Verification items for the finished model (mm, model axes). Face numbers are marked on the shaded views. Give positions to 0.01 mm unless a question says otherwise; leave off trailing zeros. Order: outer loops, then holes, each group sorted by start corner. A loop starts at its lowest first (then second) coordinate and runs counter-clockwise, first axis right, second up. Notation, with made-up numbers: (-18, 27.5) - (20, 27.5) arc R10 cw to (20, 40.5) - close; hole circle Ø5 at (-10.5, 47.5). An arc over 180 degrees is marked (long way). Answer as a JSON object with one key per item and string values. Group by question number.
(1) Thickness scan on line 1 (Y direction, x = 0, z = 17.25); line 2 (Y direction, x = -4, z = 12.25); line 3 (X direction, y = -7, z = 9.25). Record the ranges inside material, lowest first.
(2) Section check A-A (y = 0). Record the boundary of the cut face in (x, z).
(3) Mould release check, pull along X, two halves, no side actions. Record for the marked faces 1, 2 and 3: +X half, -X half, draft (parallel to the pull), parting line (faces both ways), or undercut.
(4) Section check D-D (y = -17). Record the boundary of the cut face in (x, z).
(5) Depth check by flat-ended pin: pin 1 Ø12 at (x, z) = (-4.5, 10) entering from -Y; pin 2 Ø5 at (x, z) = (-13, 3) entering from -Y; pin 3 Ø1 at (y, z) = (7, 4.5) entering from +X. Enter the tip coordinate at first touch or a pass-through.
(6) Section check C-C (z = 13). Record the boundary of the cut face in (x, y).
```python
from build123d import *

# Parameters (mm, degrees)
F0_R     = 20.9347
F1_DEPTH = 25
F2_R     = 9.210685
F3_DEPTH = 25
F4_R     = 10.317233
F5_DEPTH = 25


with BuildPart() as f1:
    # F0 (on Top) → F1 (new body)
    with BuildSketch(Plane.XY):
        Circle(F0_R)
    extrude(amount=F1_DEPTH)

    # F2 (on face) → F3 (join)
    with BuildSketch(Plane.XY.offset(25)):
        Circle(F2_R)
    extrude(amount=-F3_DEPTH)

    # F4 (on face) → F5 (cut)
    with BuildSketch(Plane.XY.offset(25)):
        Circle(F4_R)
    extrude(amount=-F5_DEPTH, mode=Mode.SUBTRACT)


solid = f1.part
```
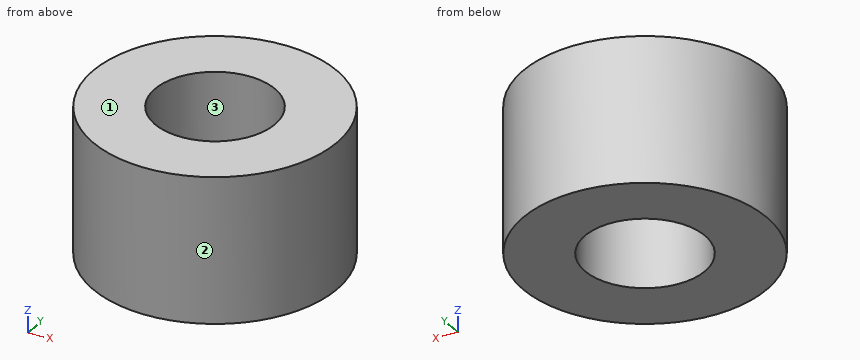
Solutions:
{
 "1": {"line 1": "y = -20.93 to -10.32, 10.32 to 20.93", "line 2": "y = -20.55 to -9.51, 9.51 to 20.55", "line 3": "x = -19.73 to -7.58, 7.58 to 19.73"},
 "2": {"outline": "(-20.93, 0) - (-10.32, 0) - (-10.32, 25) - (-20.93, 25) - close; (10.32, 0) - (20.93, 0) - (20.93, 25) - (10.32, 25) - close"},
 "3": {"face 1": "draft", "face 2": "parting line", "face 3": "undercut"},
 "4": {"outline": "(-12.22, 0) - (12.22, 0) - (12.22, 25) - (-12.22, 25) - close"},
 "5": {"pin 1": "stops at y = -20.93", "pin 2": "stops at y = -18.11", "pin 3": "stops at x = 19.9"},
 "6": {"outline": "circle Ø41.87 at (0, 0); hole circle Ø20.63 at (0, 0)"}
}
